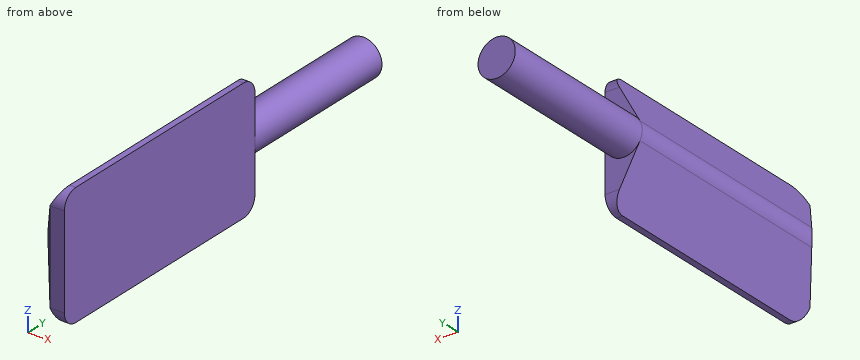
from build123d import *

# Parameters (mm, degrees)
CROQUIS1_R              = 9
SALIENTE_EXTRUIR1_DEPTH = 200
SALIENTE_EXTRUIR2_DEPTH = 120
REDONDEO1_R             = 7.2
CORTAR_EXTRUIR1_DEPTH   = 120


with BuildPart() as part:
    # Croquis1 → Saliente-Extruir1 (new body)
    with BuildSketch(Plane(origin=(0, 0, 0), x_dir=(1, 0, 0), z_dir=(0, 1, 0))):
        Circle(CROQUIS1_R)
    extrude(amount=SALIENTE_EXTRUIR1_DEPTH)

    # Croquis2 → Saliente-Extruir2 (add)
    with BuildSketch(Plane.XZ):
        with BuildLine():
            Line((6, 29.5), (-7.879793, 4.348432))
            ThreePointArc((-7.879793, 4.348432), (-9, 0), (-7.879793, -4.348432))
            Line((-7.879793, -4.348432), (6, -29.5))
            Line((6, -29.5), (9, -29.5))
            Line((9, -29.5), (9, 29.5))
            Line((9, 29.5), (6, 29.5))
        make_face()
    extrude(amount=-SALIENTE_EXTRUIR2_DEPTH)

    # Redondeo1
    redondeo1_edges = [part.edges().sort_by_distance(p)[0] for p in [
        (7.5, 0, 29.5),
        (7.5, 120, 29.5),
        (7.5, 120, -29.5),
        (7.5, 0, -29.5),
    ]]
    fillet(redondeo1_edges, radius=REDONDEO1_R)

    # Croquis3 → Cortar-Extruir1 (cut)
    with BuildSketch(Plane(origin=(0, 0, -29.5), x_dir=(-1, 0, 0), z_dir=(0, 0, -1))):
        Polygon((-2.026709, 0), (10.656807, 15.115625), (12.907476, -4.543474), align=None)
    extrude(amount=-CORTAR_EXTRUIR1_DEPTH, mode=Mode.SUBTRACT)


solid = part.part
Here's how the part is built. I have some questions about the finished solid (model axes, mm). Round coordinates to 2 decimals unless told otherwise and drop trailing zeros. Loops run counter-clockwise (first coordinate to the right, second up) from the corner with the lowest first, then second, coordinate; pieces in that order, holes last. Notation, with made-up numbers: (72.5, 68) -> (129.5, 68) arc R21 cw to (129.5, 93) -> close; hole circle Ø7 at (71.25, 58). An arc over 180 degrees is marked (long way). Write each question's results on one line, items separated by ' | '.
(1) If we section it at C-C, the plane z = -19.5: List the corners of the cut face in (x, y) for me.
Worked answers:
outline: (0.48, 1.84) -> (2.03, 0) -> (9, 0) -> (9, 120) -> (0.48, 120) -> close
(2) If I drill on L1, parallel to Y at x = 2, z = -19; L2, parallel to X at y = 35, z = 0.5; L3, parallel to X at y = 90, z = 7.5, over which ranges is the centre line in solid material (lowest first)?
Worked answers:
L1: 0.03 to 120 | L2: -8.99 to 9 | L3: -6.14 to 9
(3) If we section it at D-D, the plane y = 135: List the corners of the cut face in (x, z) for me.
Worked answers:
outline: circle Ø18 at (0, 0)
(4) For P1, Ø8, axis at x = -6, z = -3, coming from the -Y side; P2, Ø3, axis at y = 42, z = 12, coming from the -X side; P3, Ø10, axis at x = -1.5, y = 176, coming from the +Z side, each with a flat end and sliding along its axis, tell me the tip position at first contact or that it passes through.
Worked answers:
P1: y = 4.8 | P2: x = -4.49 | P3: z = 9
(5) If we section it at B-B, the plane x = -2.25: List the corners of the cut face in (y, z) for me, then the cut area to 3 significant figures.
Worked answers:
outline: (5.1, -14.55) -> (120, -14.55) -> (120, -8.71) -> (200, -8.71) -> (200, 8.71) -> (120, 8.71) -> (120, 14.55) -> (5.1, 14.55) -> close | area: 4,740 mm2
(6) If we section it at A-A, the plane y = 76: List the corners of the cut face in (x, z) for me.
Worked answers:
outline: (-7.88, -4.35) -> (6, -29.5) -> (9, -29.5) -> (9, 29.5) -> (6, 29.5) -> (-7.88, 4.35) arc R9 ccw to start
